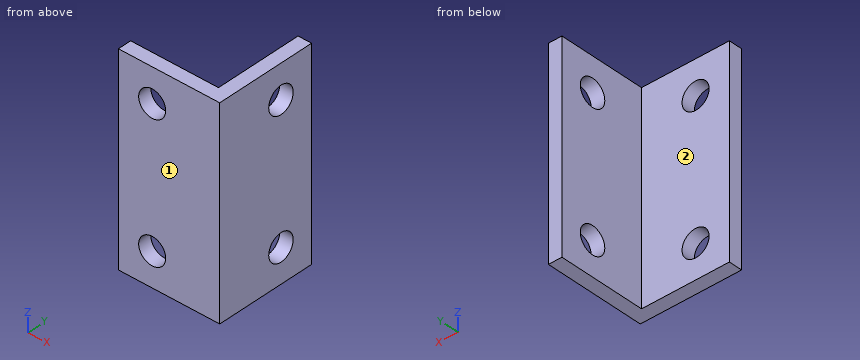
```python
from build123d import *

# Parameters (mm, degrees)
BOSS_EXTRUDE1_DEPTH = 30
CUT_EXTRUDE1_REACH  = 17
SKETCH2_R           = 2
CUT_EXTRUDE2_REACH  = 4
SKETCH3_R           = 2


with BuildPart() as part:
    # Sketch1 → Boss-Extrude1 (new body)
    with BuildSketch(Plane.XY):
        Polygon((0, 15), (0, 0), (-15, 0), (-15, 2), (-2, 2), (-2, 15), align=None)
    extrude(amount=BOSS_EXTRUDE1_DEPTH)

    # Sketch2 → Cut-Extrude1 (cut, up to next)
    with BuildSketch(Plane(origin=(0, 0, 0), x_dir=(0, 0, -1), z_dir=(1, 0, 0)), mode=Mode.PRIVATE) as cut_extrude1_sk1:
        with Locations((-25, 10)):
            Circle(SKETCH2_R)
    cut_extrude1_tool1 = extrude(cut_extrude1_sk1.sketch, amount=-CUT_EXTRUDE1_REACH, mode=Mode.PRIVATE) & part.part
    add(cut_extrude1_tool1.solids().sort_by_distance((0, 10, 25))[0], mode=Mode.SUBTRACT)
    # Sketch2 → Cut-Extrude1 (cut, up to next)
    with BuildSketch(Plane(origin=(0, 0, 0), x_dir=(0, 0, -1), z_dir=(1, 0, 0)), mode=Mode.PRIVATE) as cut_extrude1_sk2:
        with Locations((-5, 10)):
            Circle(SKETCH2_R)
    cut_extrude1_tool2 = extrude(cut_extrude1_sk2.sketch, amount=-CUT_EXTRUDE1_REACH, mode=Mode.PRIVATE) & part.part
    add(cut_extrude1_tool2.solids().sort_by_distance((0, 10, 5))[0], mode=Mode.SUBTRACT)

    # Sketch3 → Cut-Extrude2 (cut, up to next)
    with BuildSketch(Plane(origin=(0, 2, 0), x_dir=(1, 0, 0), z_dir=(0, 1, 0)), mode=Mode.PRIVATE) as cut_extrude2_sk1:
        with Locations((-10, -5)):
            Circle(SKETCH3_R)
    cut_extrude2_tool1 = extrude(cut_extrude2_sk1.sketch, amount=-CUT_EXTRUDE2_REACH, mode=Mode.PRIVATE) & part.part
    add(cut_extrude2_tool1.solids().sort_by_distance((-10, 2, 5))[0], mode=Mode.SUBTRACT)
    # Sketch3 → Cut-Extrude2 (cut, up to next)
    with BuildSketch(Plane(origin=(0, 2, 0), x_dir=(1, 0, 0), z_dir=(0, 1, 0)), mode=Mode.PRIVATE) as cut_extrude2_sk2:
        with Locations((-10, -25)):
            Circle(SKETCH3_R)
    cut_extrude2_tool2 = extrude(cut_extrude2_sk2.sketch, amount=-CUT_EXTRUDE2_REACH, mode=Mode.PRIVATE) & part.part
    add(cut_extrude2_tool2.solids().sort_by_distance((-10, 2, 25))[0], mode=Mode.SUBTRACT)


solid = part.part
```
Source: CAD feature listing. Evaluate the final solid. Frame: model axes, mm. Face numbers are marked on the shaded views. A direction names the side the tool comes from. Give positions to 0.01 mm unless a question says otherwise; leave off trailing zeros. Loops run counter-clockwise (first coordinate to the right, second up) from the corner with the lowest first, then second, coordinate; pieces in that order, holes last. Notation, with made-up numbers: (-35.75, 86.5) -> (-10.75, 86.5) arc R22 cw to (-10.75, 122.5) -> close; hole circle Ø2 at (-20.75, 0.25). An arc over 180 degrees is marked (long way). Use a Markdown table: item, result. Add a question column.
(1) Section query D-D (y = 4.75). Output: boundary loops of the cut face in (x, z).
(2) First-contact query: pin 1 Ø4.5 at (y, z) = (10, 25) entering from -X. Flat tip, straight axial feed; report the tip coordinate or a pass-through.
(3) Access query for the marked faces 1 and 2. Directions: +Z, -Z, +X, -X, +Y, -Y. A direction counts if a zero-diameter tool reaches every point of the face in a straight line with its end or side. Return the directions, or none.
(4) Section query A-A (x = -10). Output: boundary loops of the cut face in (y, z).
(5) Section query C-C (z = 12.75). Output: boundary loops of the cut face in (x, y).
(6) Ray query, line 1 (Z direction, x = -10, y = 1.2); line 2 (Y direction, x = -0.65, z = 25); line 3 (X direction, y = 1.6, z = 25). Return the intervals inside material, ascending.
(7) Section query B-B (z = 5). Output: boundary loops of the cut face in (x, y), then the cut area to 3 significant figures.
Checked values:
| question | item | result |
|---|---|---|
| 1 | outline | (-2, 0) -> (0, 0) -> (0, 30) -> (-2, 30) -> close |
| 2 | pin 1 | x = -2 |
| 3 | face 1 | +Z, -Z, +X, -X, -Y |
| 3 | face 2 | +Z, -Z, -X, +Y |
| 4 | outline | (0, 0) -> (2, 0) -> (2, 3) -> (0, 3) -> close; (0, 7) -> (2, 7) -> (2, 23) -> (0, 23) -> close; (0, 27) -> (2, 27) -> (2, 30) -> (0, 30) -> close |
| 5 | outline | (-15, 0) -> (0, 0) -> (0, 15) -> (-2, 15) -> (-2, 2) -> (-15, 2) -> close |
| 6 | line 1 | 0 to 3, 7 to 23, 27 to 30 |
| 6 | line 2 | 0 to 8, 12 to 15 |
| 6 | line 3 | -15 to -12, -8 to 0 |
| 7 | outline | (-15, 0) -> (-12, 0) -> (-12, 2) -> (-15, 2) -> close; (-8, 0) -> (0, 0) -> (0, 8) -> (-2, 8) -> (-2, 2) -> (-8, 2) -> close; (-2, 12) -> (0, 12) -> (0, 15) -> (-2, 15) -> close |
| 7 | area | 40.0 mm^2 |
